Geometry: see drawing. Coordinates: mm, zero at the bounding-box minimum. Coordinates: 2 decimals unless noted, no trailing zeros. Write each loop counter-clockwise with the first axis right and the second up, starting at its lowest first coordinate (ties: lowest second). Pieces come first, ordered by that corner, then holes.
1) Pin query (flat end, axial travel): pin 1 Ø7.5 at (y, z) = (1168.5, 8) entering from +X; pin 2 Ø8 at (y, z) = (1297.5, 8.5) entering from -X; pin 3 Ø1 at (y, z) = (242, 4.5) entering from +X. Return the tip coordinate at first contact, or that it passes through.
2) Section query C-C (x = 470.5). Output: boundary loops of the cut face in (y, z), then the cut area to 3 significant figures.
3) Line query: L1, parallel to X at y = 1339.5, z = 14; L2, parallel to X at y = 417, z = 11 (1 decimal). Output: solid intervals per line, ascending.
4) Section query A-A (z = 8). State how many separate pieces and enclosed holes the cut face has, then the cut area to 3 significant figures.
5) Section query B-B (x = 271). Output: boundary loops of the cut face in (y, z) (1 decimal), then the cut area to 3 significant figures.
6) Section query D-D (y = 387). Output: boundary loops of the cut face in (x, z).
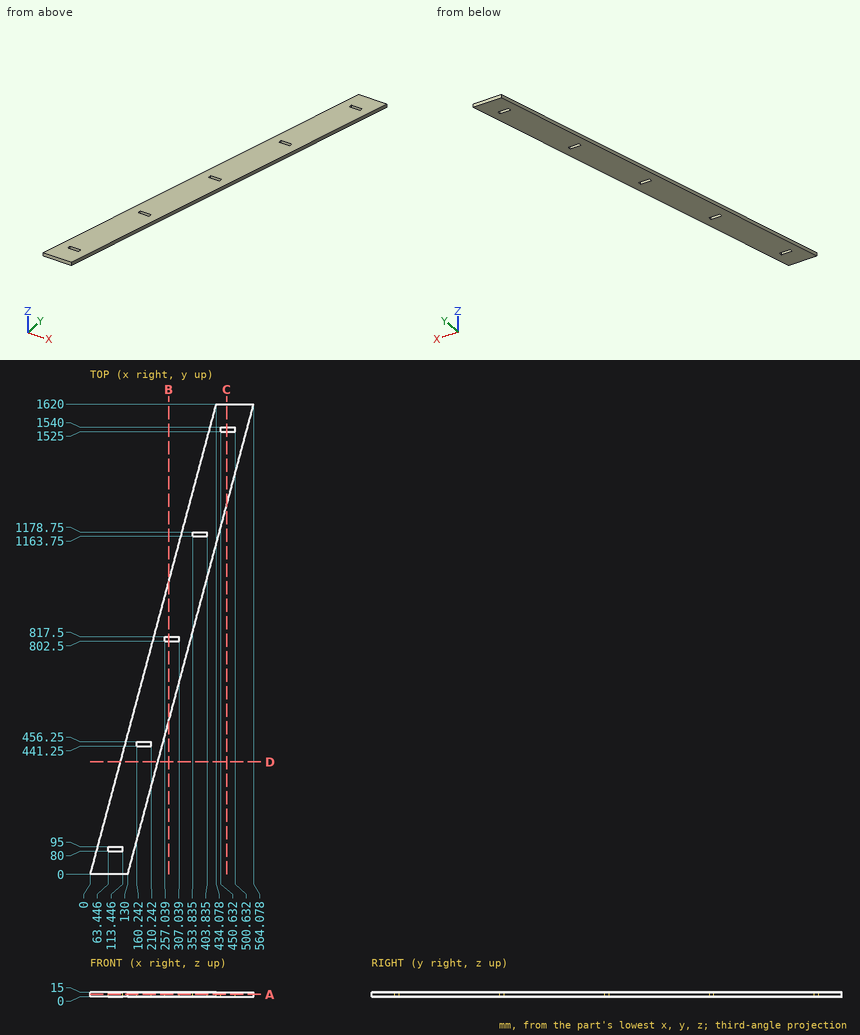
Answer:
1. pin 1: stops at x = 444.1
1. pin 2: stops at x = 346.59
1. pin 3: stops at x = 194.98
2. outline: (1270.76, 0) - (1525, 0) - (1525, 15) - (1270.76, 15) - close; (1540, 0) - (1620, 0) - (1620, 15) - (1540, 15) - close
2. area: 5,010 mm2
3. L1: x = 358.92 to 488.92
3. L2: x = 111.7 to 241.7
4. separate pieces: 1
4. enclosed holes: 5
4. area: 207,000 mm2
5. outline: (526.2, 0) - (802.5, 0) - (802.5, 15) - (526.2, 15) - close; (817.5, 0) - (1011.4, 0) - (1011.4, 15) - (817.5, 15) - close
5. area: 7,050 mm2
6. outline: (103.7, 0) - (233.7, 0) - (233.7, 15) - (103.7, 15) - close
